```python
from build123d import *

# Parameters (mm, degrees)
SKETCH1_W           = 188.9
SKETCH1_H           = 158.9
BOSS_EXTRUDE1_DEPTH = 5
SKETCH2_W           = 170
SKETCH2_H           = 140
CUT_EXTRUDE1_DEPTH  = 1.66
SKETCH3_R           = 1.65
CUT_EXTRUDE2_DEPTH  = 5
SKETCH6_R           = 1.65
CUT_EXTRUDE4_DEPTH  = 10
SKETCH7_R           = 1.75
CUT_EXTRUDE5_DEPTH  = 10


with BuildPart() as part:
    # Sketch1 → Boss-Extrude1 (new body)
    with BuildSketch(Plane(origin=(0, 0, 0), x_dir=(1, 0, 0), z_dir=(0, 1, 0))):
        Rectangle(SKETCH1_W, SKETCH1_H)
    extrude(amount=BOSS_EXTRUDE1_DEPTH)

    # Sketch2 → Cut-Extrude1 (cut)
    with BuildSketch(Plane(origin=(0, 5, 0), x_dir=(1, 0, 0), z_dir=(0, 1, 0))):
        Rectangle(SKETCH2_W, SKETCH2_H)
    extrude(amount=-CUT_EXTRUDE1_DEPTH, mode=Mode.SUBTRACT)

    # Sketch3 → Cut-Extrude2 (cut)
    with BuildSketch(Plane(origin=(0, 5, 0), x_dir=(1, 0, 0), z_dir=(0, 1, 0))):
        with Locations((-90, 75)):
            Circle(SKETCH3_R)
    extrude(amount=-CUT_EXTRUDE2_DEPTH, mode=Mode.SUBTRACT)

    # Sketch6 → Cut-Extrude4 (cut)
    with BuildSketch(Plane(origin=(0, 5, 0), x_dir=(1, 0, 0), z_dir=(0, 1, 0))):
        with Locations((-90, -75)):
            Circle(SKETCH6_R)
        with Locations((89.9, -75)):
            Circle(SKETCH6_R)
        with Locations((90, 75)):
            Circle(SKETCH6_R)
    extrude(amount=-CUT_EXTRUDE4_DEPTH, mode=Mode.SUBTRACT)

    # Sketch7 → Cut-Extrude5 (cut)
    with BuildSketch(Plane(origin=(0, 3.34, 0), x_dir=(1, 0, 0), z_dir=(0, 1, 0))):
        with Locations((-74.352299287, 62.544099294)):
            Circle(SKETCH7_R)
        with Locations((74.352299287, -62.544099294)):
            Circle(SKETCH7_R)
        with Locations((-59.047144008, 49.669619814)):
            Circle(SKETCH7_R)
        with Locations((-43.741988729, 36.795140334)):
            Circle(SKETCH7_R)
        with Locations((-28.43683345, 23.920660853)):
            Circle(SKETCH7_R)
        with Locations((-13.131678171, 11.046181373)):
            Circle(SKETCH7_R)
        with Locations((13.131678171, 11.046181373)):
            Circle(SKETCH7_R)
        with Locations((28.43683345, 23.920660853)):
            Circle(SKETCH7_R)
        with Locations((43.741988729, 36.795140334)):
            Circle(SKETCH7_R)
        with Locations((59.047144008, 49.669619814)):
            Circle(SKETCH7_R)
        with Locations((74.352299287, 62.544099294)):
            Circle(SKETCH7_R)
        with Locations((59.047144008, -49.669619814)):
            Circle(SKETCH7_R)
        with Locations((43.741988729, -36.795140334)):
            Circle(SKETCH7_R)
        with Locations((28.43683345, -23.920660853)):
            Circle(SKETCH7_R)
        with Locations((13.131678171, -11.046181373)):
            Circle(SKETCH7_R)
        with Locations((-13.131678171, -11.046181373)):
            Circle(SKETCH7_R)
        with Locations((-28.43683345, -23.920660853)):
            Circle(SKETCH7_R)
        with Locations((-43.741988729, -36.795140334)):
            Circle(SKETCH7_R)
        with Locations((-59.047144008, -49.669619814)):
            Circle(SKETCH7_R)
        with Locations((-74.352299287, -62.544099294)):
            Circle(SKETCH7_R)
    extrude(amount=-CUT_EXTRUDE5_DEPTH, mode=Mode.SUBTRACT)


solid = part.part
```
Verification items for the finished model (mm, model axes). A direction names the side the tool comes from. Round coordinates to 2 decimals unless told otherwise and drop trailing zeros. Write each loop counter-clockwise with the first axis right and the second up, starting at its lowest first coordinate (ties: lowest second). Pieces come first, ordered by that corner, then holes. Notation, with made-up numbers: (-36.75, 49) - (-23.75, 49) arc R25 cw to (-23.75, 74) - close; hole circle Ø1 at (-14, 60.5). An arc over 180 degrees is marked (long way). Answer as a JSON object with one key per item and string values. Group by question number.
Q1. Section check A-A, the plane y = 4.1. Enter the section's corners in (x, z).
Q2. Tool access check on faces 1 (the flat face through (-1, 2, 79.45)), 2 (the flat face through (-1, 3.34, -1)). Record the directions out of +Z, -Z, +X, -X, +Y, -Y that give a thin tool (end or side, any length) a straight path to the whole face; none if there is none.
Q3. Thickness scan on line 1 (Z direction, x = 89.9, y = 1.2); line 2 (X direction, y = 0.7, z = 63.5); line 3 (X direction, y = 1.1, z = 38). Record the ranges inside material, lowest first.
Q4. Section check C-C, the plane z = 6. Enter the section's corners in (x, y), plus the area to 3 significant figures.
Q5. Go/stop test with flat-tipped pins: pin 1 Ø4 at (x, z) = (-74.35, 62.54) entering from +Y; pin 2 Ø8 at (x, z) = (47.5, 42.5) entering from -Y. Record where each tip stops, or that it passes through.
Q6. Section check B-B, the plane x = -81.5. Enter the section's corners in (y, z).
Found:
{
 "1": {"outline": "(-94.45, -79.45) - (94.45, -79.45) - (94.45, 79.45) - (-94.45, 79.45) - close; hole circle Ø3.3 at (-90, -75); hole circle Ø3.3 at (-90, 75); hole (-85, -70) - (85, -70) - (85, 70) - (-85, 70) - close; hole circle Ø3.3 at (89.9, 75); hole circle Ø3.3 at (90, -75)"},
 "2": {"face 1": "+Z, +X, -X, +Y, -Y", "face 2": "+Y"},
 "3": {"line 1": "z = -79.45 to -76.65, -73.35 to 73.35, 76.65 to 79.45", "line 2": "x = -94.45 to -75.82, -72.89 to 72.89, 75.82 to 94.45", "line 3": "x = -94.45 to -45.01, -42.47 to 42.47, 45.01 to 94.45"},
 "4": {"outline": "(-94.45, 0) - (94.45, 0) - (94.45, 5) - (85, 5) - (85, 3.34) - (-85, 3.34) - (-85, 5) - (-94.45, 5) - close", "area": "662 mm^2"},
 "5": {"pin 1": "stops at y = 3.34", "pin 2": "stops at y = 0"},
 "6": {"outline": "(0, -79.45) - (5, -79.45) - (5, -70) - (3.34, -70) - (3.34, 70) - (5, 70) - (5, 79.45) - (0, 79.45) - close"}
}
